Source: CAD feature listing. Evaluate the final solid. Frame: model axes, mm. A direction names the side the tool comes from. Round coordinates to 2 decimals unless told otherwise and drop trailing zeros. Order: outer loops, then holes, each group sorted by start corner. A loop starts at its lowest first (then second) coordinate and runs counter-clockwise, first axis right, second up. Notation, with made-up numbers: (56, -30) - (71, -30) arc R24 ccw to (71, -9) - close; hole circle Ø7 at (-5, 31). An arc over 180 degrees is marked (long way). Return JSON: item names as keys, results as strings. Group by question number.
1) Contact query for flat-ended pins moving along their axis: P1, Ø12.5, axis at y = -9, z = 33.5, coming from the -X side; P2, Ø2, axis at x = 37.5, z = 40, coming from the -Y side; P3, Ø15, axis at x = -2.5, z = -10.5, coming from the -Y side. Output: stop coordinate, or through.
2) Ray query, line 1 (X direction, y = -45, z = -15); line 2 (X direction, y = -17, z = 28.5); line 3 (Z direction, x = -41, y = -44). Return the intervals inside material, ascending. Write a range as from..to.
3) Access query for faces 4 (the flat face through (-1, -30, -30)), 5 (the flat face through (1, -25, 25)), 6 (the flat face through (18, -47, -15)). Directions: +Z, -Z, +X, -X, +Y, -Y. A direction counts if a zero-diameter tool reaches every point of the face in a straight line with its end or side. Return the directions, or none.
4) Section A-A, the plane z = 25. Return loops of the section in (x, y).
5) Mould query, pull axis X, two halves, no side actions, for faces 1 (the flat face through (-54.933, -12, 25)), 2 (the flat face through (36, -60, -15)), 3 (the cylindrical face through (32.46, -12.32, 28.06)). Classes: pulls with the +X half, pulls with the -X half, needs draft (parallel to the pull), parting line crosses it, or undercut.
6) Section B-B, the plane y = -49.5. Return loops of the section in (x, z).
7) Section D-D, the plane y = -11.5. Return loops of the section in (x, z).
8) Section C-C, the plane x = -20. Return loops of the section in (y, z).
Solid Edge part; units mm, degrees
sketch "Sketch1" plane through (0, 0, 0) normal (0, 0, 1) x (1, 0, 0)
  line L0 (55, -60) -> (55, 0)
  line L1 (55, 0) -> (-55, 0)
  line L2 (-55, 0) -> (-55, -60)
  line L3 (-55, -60) -> (-22, -60)
  line L4 (-22, -60) -> (-22, -35)
  line L5 (-22, -35) -> (18, -35)
  line L6 (18, -35) -> (18, -60)
  line L7 (18, -60) -> (55, -60)
extrude "Protrusion1" add sketch "Sketch1" against normal blind 30
sketch "Sketch2" plane through (0, 0, 0) normal (0, -1, 0) x (1, 0, 0)
  circle A0 centre (-24.9329, 25) radius 8
  circle A1 centre (25.0671, 25) radius 8
  line L0 (-54.9329, 0) -> (55, 0)
  line L1 (55, 0) -> (55, 50)
  line L2 (55, 50) -> (-54.9329, 50)
  line L3 (-54.9329, 50) -> (-54.9329, 0)
extrude "ExtrudedProtrusion_2" add sketch "Sketch2" along normal blind 25
Geometry check:
{
 "1": {"P1": "x = -54.93", "P2": "y = -25", "P3": "y = -35"},
 "2": {"line 1": "-55..-22, 18..55", "line 2": "-54.93..-32.13, -17.74..17.87, 32.26..55", "line 3": "-30..0"},
 "3": {"face 4": "-Z, +X, -X, +Y, -Y", "face 5": "+Z, +X, -X, -Y", "face 6": "+Z, -Z, -Y"},
 "4": {"outline": "(-54.93, -25) - (-32.93, -25) - (-32.93, 0) - (-54.93, 0) - close; (-16.93, -25) - (17.07, -25) - (17.07, 0) - (-16.93, 0) - close; (33.07, -25) - (55, -25) - (55, 0) - (33.07, 0) - close"},
 "5": {"face 1": "pulls with the -X half", "face 2": "needs draft", "face 3": "undercut"},
 "6": {"outline": "(-55, -30) - (-22, -30) - (-22, 0) - (-55, 0) - close; (18, -30) - (55, -30) - (55, 0) - (18, 0) - close"},
 "7": {"outline": "(-55, -30) - (55, -30) - (55, 50) - (-54.93, 50) - (-54.93, 0) - (-55, 0) - close; hole circle Ø16 at (-24.93, 25); hole circle Ø16 at (25.07, 25)"},
 "8": {"outline": "(-35, -30) - (0, -30) - (0, 18.7) - (-25, 18.7) - (-25, 0) - (-35, 0) - close; (-25, 31.3) - (0, 31.3) - (0, 50) - (-25, 50) - close"}
}
